Read the model definition and answer for the solid it produces. Units are mm, in the model's axes. A direction names the side the tool comes from. Coordinates: 2 decimals unless noted, no trailing zeros. Loops run counter-clockwise (first coordinate to the right, second up) from the corner with the lowest first, then second, coordinate; pieces in that order, holes last.
from build123d import *

# Parameters (mm, degrees)
SKETCH3_R           = 12.2
SKETCH3_R_2         = 3.2
BOSS_EXTRUDE1_DEPTH = 49.8
SKETCH4_R           = 3.5
SKETCH4_R_2         = 2
BOSS_EXTRUDE2_DEPTH = 2.38


with BuildPart() as part:
    # Sketch3 → Boss-Extrude1 (new body)
    with BuildSketch(Plane(origin=(0, 0, 0), x_dir=(1, 0, 0), z_dir=(0, 1, 0))):
        Circle(SKETCH3_R)
        Circle(SKETCH3_R_2, mode=Mode.SUBTRACT)
    extrude(amount=BOSS_EXTRUDE1_DEPTH)

    # Sketch4 → Boss-Extrude2 (add)
    with BuildSketch(Plane(origin=(0, 49.8, 0), x_dir=(1, 0, 0), z_dir=(0, 1, 0))):
        Circle(SKETCH4_R)
        Circle(SKETCH4_R_2, mode=Mode.SUBTRACT)
    extrude(amount=BOSS_EXTRUDE2_DEPTH)


solid = part.part
Q1. A cutting plane is placed at C-C (y = 15.5). Give the vertices of the cut face in (x, z), then the cut area to 3 significant figures.
Findings below:
outline: circle Ø24.4 at (0, 0); hole circle Ø6.4 at (0, 0)
area: 435 mm2
Q2. Determine the mould class of faces 1 (the face through (3, 49.8, 3)), 2 (the face through (2, 49.8, 1)), 3 (the face through (-12.19, 24.55, -0.54)) for opening direction X: +X half, -X half, draft (parallel to the pull), parting line (faces both ways), or undercut.
Findings below:
face 1: draft
face 2: undercut
face 3: parting line
Q3. Straight lines are drawn through the part: probe 1 along Z at (x, y) = (0, 51.35); probe 2 along X at (y, z) = (20, 0). For each, find the intervals that lie inside material, in ascending order.
Findings below:
probe 1: z = -3.5 to -2, 2 to 3.5
probe 2: x = -12.2 to -3.2, 3.2 to 12.2
Q4. Which of the six approach directions +Z, -Z, +X, -X, +Y, -Y give full straight-line access (tool end or side, diameter ignored) to faces 4 (the face through (-2.539, 24.551, 1.947)), 5 (the face through (2, 52.18, 2)), 6 (the face through (3.233, 50.973, 1.341))?
Findings below:
face 4: -Y
face 5: +Z, -Z, +X, -X, +Y
face 6: +Y
Q5. A cutting plane is placed at D-D (z = -7.75). Give the vertices of the cut face in (x, y), then the cut area to 3 significant figures.
Findings below:
outline: (-9.42, 0) - (9.42, 0) - (9.42, 49.8) - (-9.42, 49.8) - close
area: 938 mm2
Q6. A cutting plane is placed at B-B (x = 0). Give the vertices of the cut face in (y, z).
Findings below:
outline: (0, -12.2) - (49.8, -12.2) - (49.8, -3.5) - (52.18, -3.5) - (52.18, -2) - (49.8, -2) - (49.8, -3.2) - (0, -3.2) - close; (0, 3.2) - (49.8, 3.2) - (49.8, 2) - (52.18, 2) - (52.18, 3.5) - (49.8, 3.5) - (49.8, 12.2) - (0, 12.2) - close
Q7. A cutting plane is placed at A-A (z = 0). Give the vertices of the cut face in (x, y).
Findings below:
outline: (-12.2, 0) - (-3.2, 0) - (-3.2, 49.8) - (-2, 49.8) - (-2, 52.18) - (-3.5, 52.18) - (-3.5, 49.8) - (-12.2, 49.8) - close; (2, 49.8) - (3.2, 49.8) - (3.2, 0) - (12.2, 0) - (12.2, 49.8) - (3.5, 49.8) - (3.5, 52.18) - (2, 52.18) - close
Q8. Flat-ended cylindrical pins translate along their axes: pin 1 Ø3 at (x, y) = (-3.5, 34) entering from +Z; pin 2 Ø7 at (x, z) = (-1, -0.5) entering from -Y; pin 3 Ø4 at (x, y) = (-3.5, 24.5) entering from -Z; pin 4 Ø12 at (y, z) = (12.5, -9.5) entering from +X. Find the tip coordinate at first contact, or state that the pin passes through.
Findings below:
pin 1: stops at z = 12.03
pin 2: stops at y = 0
pin 3: stops at z = -12.11
pin 4: stops at x = 11.69
